```python
from build123d import *

# Parameters (mm, degrees)
BOSS_EXTRUDE1_START     = -40
BOSS_EXTRUDE1_OUTLINE_R = 5
BOSS_EXTRUDE1_DEPTH     = 40
CUT_EXTRUDE1_DEPTH      = 2
BOSS_EXTRUDE2_DEPTH     = 3
FILLET1_R               = 3


# Read off the part's stored shape, not the designer's step: Boss-Extrude1
with BuildPart() as part:
    # Boss-Extrude1 outline → Boss-Extrude1 (new body)
    with BuildSketch(Plane.XZ.offset(-110).offset(BOSS_EXTRUDE1_START)):
        Circle(BOSS_EXTRUDE1_OUTLINE_R)
    extrude(amount=BOSS_EXTRUDE1_DEPTH)

    # Sketch12 → Cut-Extrude1 (cut)
    with BuildSketch(Plane(origin=(0, 150, 0), x_dir=(1, 0, 0), z_dir=(0, 1, 0))):
        with BuildLine():
            Line((1.5, -4.769696007), (1.5, 4.769696007))
            ThreePointArc((1.5, 4.769696007), (0, 5), (-1.5, 4.769696007))
            Line((-1.5, 4.769696007), (-1.5, -4.769696007))
            ThreePointArc((-1.5, -4.769696007), (0, -5), (1.5, -4.769696007))
        make_face()
    extrude(amount=-CUT_EXTRUDE1_DEPTH, mode=Mode.SUBTRACT)

    # Sketch13 → Boss-Extrude2 (add)
    with BuildSketch(Plane(origin=(0, 150, 0), x_dir=(1, 0, 0), z_dir=(0, 1, 0))):
        with BuildLine():
            Line((1.5, 5.473173211), (1.5, -5.473173211))
            ThreePointArc((1.5, -5.473173211), (6.3, 0), (1.5, 5.473173211))
        make_face()
        with BuildLine():
            Line((-1.5, 5.473173211), (-1.5, -5.473173211))
            ThreePointArc((-1.5, -5.473173211), (-6.3, 0), (-1.5, 5.473173211))
        make_face()
    extrude(amount=BOSS_EXTRUDE2_DEPTH)

    # Fillet1
    fillet1_edges = [part.edges().sort_by_distance(p)[0] for p in [
        (-6.3, 153, 0),
        (6.3, 153, 0),
    ]]
    fillet(fillet1_edges, radius=FILLET1_R - 0.0001)  # a hair under: the kernel refuses the full size


solid = part.part
```
Could you check a few things on this model? Use its own coordinates, in mm. A direction names the side the tool comes from. Round coordinates to 2 decimals unless told otherwise and drop trailing zeros. Loops run counter-clockwise (first coordinate to the right, second up) from the corner with the lowest first, then second, coordinate; pieces in that order, holes last. Notation, with made-up numbers: (74, -24.5) - (81, -24.5) arc R22 cw to (81, 0.5) - close; hole circle Ø8 at (42, 27.5). An arc over 180 degrees is marked (long way). Answer in a Markdown table with one row per item. Add a question column.
(1) If we section it at A-A (y = 124): Please give me the cut outline in (x, z), plus the area to 3 significant figures.
(2) If we section it at B-B (x = 0): Please give me the cut outline in (y, z).
(3) I'm going to push flat-ended pins straight in: pin 1 (1.5 mm diameter, centred on x = -4.5, z = -4, fed in from -Y); pin 2 (2.5 mm diameter, centred on y = 151, z = 2, fed in from -X); pin 3 (1.5 mm diameter, centred on x = -2.5, y = 139.5, fed in from +Z). Where does each tip first touch, or does it pass through?
(4) For faces 1 (the face through (-5.3, 150, 0.4)), 2 (the face through (1.5, 150, 0)), 3 (the face through (0, 110, 0)), 4 (the face through (5.3, 150, 0.4)), 5 (the face through (4.77, 130.28, 1.5)), which set-ups out of +Z, -Z, +X, -X, +Y, -Y let a thin tool reach every point of the face, with its end or its side?
(5) I need wall thicknesses on line 1 along Y through (x, z) = (3.5, -0.5); line 2 along Y through (x, z) = (-0.75, -3.75); line 3 along X through (y, z) = (118, 0). Which ranges of each line are inside material? Lowest first, please.
Model answer:
| question | item | result |
|---|---|---|
| 1 | outline | circle Ø10 at (0, 0) |
| 1 | area | 78.5 mm² |
| 2 | outline | (110, -5) - (148, -5) - (148, 5) - (110, 5) - close |
| 3 | pin 1 | stops at y = 150 |
| 3 | pin 2 | stops at x = -6.2 |
| 3 | pin 3 | stops at z = 4.68 |
| 4 | face 1 | -X, -Y |
| 4 | face 2 | +Z, -Z, +Y |
| 4 | face 3 | +Z, -Z, +X, -X, -Y |
| 4 | face 4 | +X, -Y |
| 4 | face 5 | -Y |
| 5 | line 1 | y = 110 to 152.99 |
| 5 | line 2 | y = 110 to 148 |
| 5 | line 3 | x = -5 to 5 |
